Read the model definition and answer for the solid it produces. Units are mm, in the model's axes. A direction names the side the tool comes from. Coordinates: 2 decimals unless noted, no trailing zeros. Order: outer loops, then holes, each group sorted by start corner. A loop starts at its lowest first (then second) coordinate and runs counter-clockwise, first axis right, second up. Notation, with made-up numbers: M 30.25,85 L 79.25,85 A24 cw 79.25,100 Z; hole C -22,73 d6. An arc over 180 degrees is marked long. Put each result on its own line as item: value.
Autodesk Inventor part; units mm, degrees
ref_plane "YZ Plane" through (0, 0, 0) normal (1, 0, 0) x (0, 1, 0)
ref_plane "XZ Plane" through (0, 0, 0) normal (0, 1, 0) x (-1, 0, 0)
ref_plane "XY Plane" through (0, 0, 0) normal (0, 0, 1) x (1, 0, 0)
sketch "スケッチ1" plane through (0, 0, 0) normal (0, 0, 1) x (1, 0, 0)
  line L0 (0, 0) -> (40, 0)
  line L1 (40, 0) -> (40, 10)
  line L2 (40, 10) -> (0, 10)
  line L3 (0, 10) -> (0, 0)
  line L4 (12.5, 17.5) -> (27.5, 17.5)
  line L5 (27.5, 17.5) -> (27.5, 10)
  line L6 (27.5, 10) -> (12.5, 10)
  line L7 (12.5, 10) -> (12.5, 17.5)
  line L8 (0, 17.5) -> (40, 17.5)
  line L9 (40, 17.5) -> (40, 27.5)
  line L10 (40, 27.5) -> (0, 27.5)
  line L11 (0, 27.5) -> (0, 17.5)
  circle A0 centre (5, 5) radius 2
  circle A1 centre (35, 5) radius 2
  circle A2 centre (5, 22.5) radius 2
  circle A3 centre (35, 22.5) radius 2
  point P0 (40, 22.5)
  point P1 (0, 5)
  point P2 (40, 5)
  point P3 (20, 17.5)
  point P4 (12.5, 20)
  point P5 (27.5, 20)
  dimension "d0" = 40
  dimension "d1" = 10
  dimension "d2" = 7.5
  dimension "d3" = 15
  dimension "d4" = 12.5
  dimension "d5" = 40
  dimension "d6" = 10
  dimension "d8" = 12.5
  dimension "d9" = 4
  dimension "d10" = 4
  dimension "d11" = 4
  dimension "d12" = 4
  dimension "d16" = 5
  dimension "d17" = 5
  dimension "d25" = 7.5
extrude "押し出し1" add sketch "スケッチ1" along normal blind 3
fillet "フィレット1" radius 2 12 edges at (40, 27.5, 1.5) (40, 17.5, 1.5) (0, 27.5, 1.5) (0, 17.5, 1.5) (12.5, 17.5, 1.5) (27.5, 17.5, 1.5) (27.5, 10, 1.5) (40, 10, 1.5) (40, 0, 1.5) (12.5, 10, 1.5) (0, 10, 1.5) (0, 0, 1.5)
equation "\"d8\" = d4"
properties part number "mountT"
Q1. For a pull along X with two mould halves and no side action, classify faces 1 (the face through (0.57, 18.1, 1.52)), 2 (the face through (28.07, 10.6, 1.52)), 3 (the face through (36.908, 21.899, 1.479)) as +X half, -X half, draft (parallel to the pull), parting line (faces both ways), or undercut.
Answers below:
face 1: -X half
face 2: +X half
face 3: undercut
Q2. Consider line 1 along Y through (x, z) = (5, 1.9); line 2 along X through (y, z) = (13.75, 1.05); line 3 along Y through (x, z) = (10, 0.7). Determine where each line is inside the solid, lowest interval first.
Answers below:
line 1: y = 0 to 3, 7 to 10, 17.5 to 20.5, 24.5 to 27.5
line 2: x = 12.5 to 27.5
line 3: y = 0 to 10, 17.5 to 27.5
Q3. Given pin 1 (1.5 mm diameter, centred on y = 14.5, z = 2, fed in from -X), flat-ended and moving along its own axis, determine where the tip first touches the part or whether it passes through.
Answers below:
pin 1: stops at x = 12.5
Q4. Find section C-C on y = 5. Write down the section's boundary in (x, z), plus the area to 3 significant figures.
Answers below:
outline: M 0,0 L 3,0 L 3,3 L 0,3 Z; M 7,0 L 33,0 L 33,3 L 7,3 Z; M 37,0 L 40,0 L 40,3 L 37,3 Z
area: 96.0 mm^2
Q5. Find section A-A on z = 2.6. Write down the section's boundary in (x, y).
Answers below:
outline: M 0,2 A2 ccw 2,0 L 38,0 A2 ccw 40,2 L 40,8 A2 ccw 38,10 L 29.5,10 A2 cw 27.5,12 L 27.5,15.5 A2 cw 29.5,17.5 L 38,17.5 A2 ccw 40,19.5 L 40,25.5 A2 ccw 38,27.5 L 2,27.5 A2 ccw 0,25.5 L 0,19.5 A2 ccw 2,17.5 L 10.5,17.5 A2 cw 12.5,15.5 L 12.5,12 A2 cw 10.5,10 L 2,10 A2 ccw 0,8 Z; hole C 5,5 d4; hole C 5,22.5 d4; hole C 35,5 d4; hole C 35,22.5 d4
Q6. Find section D-D on x = 31. Write down the section's boundary in (y, z), plus the area to 3 significant figures.
Answers below:
outline: M 0,0 L 10,0 L 10,3 L 0,3 Z; M 17.5,0 L 27.5,0 L 27.5,3 L 17.5,3 Z
area: 60.0 mm^2
Q7. A tool of negligible diameter and unlimited length cuts with its end or side. For faces 4 (the face through (34, 17.5, 1)), 5 (the face through (0.6, 26.93, 1.52)), 6 (the face through (12.5, 14, 1)), from which of +Z, -Z, +X, -X, +Y, -Y can it reach the whole face along a straight path? Write none if from no direction.
Answers below:
face 4: +Z, -Z, +X
face 5: +Z, -Z, -X, +Y
face 6: +Z, -Z, -X
Q8. Find section B-B on x = 35. Write down the section's boundary in (y, z), plus the area to 3 significant figures.
Answers below:
outline: M 0,0 L 3,0 L 3,3 L 0,3 Z; M 7,0 L 10,0 L 10,3 L 7,3 Z; M 17.5,0 L 20.5,0 L 20.5,3 L 17.5,3 Z; M 24.5,0 L 27.5,0 L 27.5,3 L 24.5,3 Z
area: 36.0 mm^2
